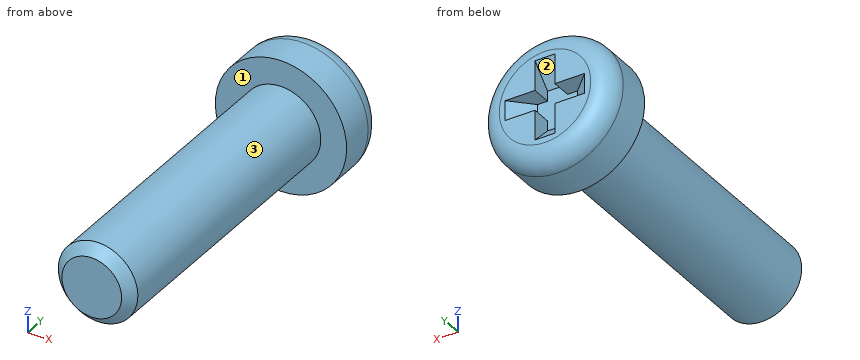
from build123d import *

# Parameters (mm, degrees)
SKETCH_1_R          = 2
EXTRUDE_1_DEPTH     = 15
SKETCH_2_R          = 3.3
EXTRUDE_2_DEPTH     = 2.7
FILLET_1_R          = 1
CHAMFER_1_SIZE      = 0.5
SKETCH_3_W          = 4
SKETCH_3_H          = 1
SKETCH_3_W_2        = 1
SKETCH_3_H_2        = 4
CUT_EXTRUDE_1_DEPTH = 1
CHAMFER_2_SIZE      = 1


with BuildPart() as part:
    # 草图1 → 凸台-拉伸1 (new body)
    with BuildSketch(Plane(origin=(0, 0, 0), x_dir=(1, 0, 0), z_dir=(0, 1, 0))):
        with Locations(Location((0, 0, 0), (0, 0, 270))):
            Circle(SKETCH_1_R)
    extrude(amount=EXTRUDE_1_DEPTH)

    # 草图2 → 凸台-拉伸2 (add)
    with BuildSketch(Plane(origin=(0, 15, 0), x_dir=(1, 0, 0), z_dir=(0, 1, 0))):
        with Locations(Location((0, 0, 0), (0, 0, 90))):
            Circle(SKETCH_2_R)
    extrude(amount=EXTRUDE_2_DEPTH)

    # 圆角1
    fillet_1_edges = [part.edges().sort_by_distance(p)[0] for p in [
        (0, 17.7, 3.3),
    ]]
    fillet(fillet_1_edges, radius=FILLET_1_R)

    # 倒角1
    chamfer_1_edges = [part.edges().sort_by_distance(p)[0] for p in [
        (0, 0, -2),
    ]]
    chamfer(chamfer_1_edges, length=CHAMFER_1_SIZE)

    # 草图3 → 切除-拉伸-薄壁1 (cut)
    with BuildSketch(Plane(origin=(0, 17.7, 0), x_dir=(1, 0, 0), z_dir=(0, 1, 0))):
        Rectangle(SKETCH_3_W, SKETCH_3_H)
        Rectangle(SKETCH_3_W_2, SKETCH_3_H_2)
    extrude(amount=-CUT_EXTRUDE_1_DEPTH, mode=Mode.SUBTRACT)

    # 倒角2
    chamfer_2_edges = [part.edges().sort_by_distance(p)[0] for p in [
        (0, 16.7, 2),
        (2, 16.7, 0),
        (0, 16.7, -2),
        (-2, 16.7, 0),
    ]]
    chamfer(chamfer_2_edges, length=CHAMFER_2_SIZE - 0.0001)  # a hair under: the kernel refuses the full size


solid = part.part
Input: part model. Units: mm. Frame: model coordinates. Face numbers are marked on the shaded views. Coordinates: 2 decimals unless noted, no trailing zeros. Order: outer loops, then holes, each group sorted by start corner. A loop starts at its lowest first (then second) coordinate and runs counter-clockwise, first axis right, second up. Notation, with made-up numbers: M 65.5,43.5 L 111.5,43.5 A12 cw 111.5,56.5 Z; hole C 80.25,85 d8. An arc over 180 degrees is marked long. Write item = value, one per line. Start each with the question number.
(1) Line query: line 1 along Y through (x, z) = (-0.25, 0.5); line 2 along Y through (x, z) = (2.25, 0.75); line 3 along Z through (x, y) = (-0.25, 13.5). Output: solid intervals per line, ascending. Write a range as [from, to].
(2) First-contact query: P1, Ø1.1, axis at x = -1.5, y = 17.5, coming from the -Z side; P2, Ø1.1, axis at x = -1.5, y = 17.5, coming from the +Z side; P3, Ø0.8, axis at y = 17, z = 1, coming from the -X side. Flat tips, straight axial feed; report the tip coordinate or a pass-through.
(3) Section C-C on y = 14. Output: boundary loops of the cut face in (x, z).
(4) Pull-direction query (X, two-part tool) for the marked faces 1, 2 and 3; classes: released by +X, released by -X, zero draft, split by the parting line, or undercut.
Result set:
q1.line_1 = [0, 16.7]
q1.line_2 = [15, 17.7]
q1.line_3 = [-1.98, 1.98]
q2.P1 = -3.01
q2.P2 = 3.01
q2.P3 = -3.23
q3.outline = C 0,0 d4
q4.face_1 = zero draft
q4.face_2 = undercut
q4.face_3 = split by the parting line
